Geometry check sheet. Reference: the model listing, model coordinates, mm. A direction names the side the tool comes from. Round coordinates to 2 decimals unless told otherwise and drop trailing zeros. Write each loop counter-clockwise with the first axis right and the second up, starting at its lowest first coordinate (ties: lowest second). Pieces come first, ordered by that corner, then holes.
Item 1: Access from +Z, -Z, +X, -X, +Y, -Y to the whole of each face (thin tool, end or side, straight path). Record for faces 1 (the face through (0, -115, 56)), 2 (the face through (3, -115, 54)).
Item 2: Cross-section at B-B (z = 31). Enter the section's corners in (x, y), then the cut area to 3 significant figures.
Item 3: Cross-section at A-A (y = -113.5). Enter the section's corners in (x, z).
Item 4: Cross-section at D-D (z = 52). Enter the section's corners in (x, y), then the cut area to 3 significant figures.
Item 5: Depth check by flat-ended pin: P1, Ø6, axis at x = 145, z = 97.5, coming from the +Y side; P2, Ø12, axis at x = 137, y = -119, coming from the -Z side. Enter the tip coordinate at first touch or a pass-through.
Item 6: Scan lines: probe 1 along Z at (x, y) = (2, -113.5); probe 2 along Y at (x, z) = (19.5, 89); probe 3 along X at (y, z) = (-25, 29). Record each from-to range of solid material in increasing order.
Item 7: Draft check along Z on faces 3 (the face through (98, 0, 54)), 4 (the face through (1.479, -102.444, 41.138)), 5 (the face through (98, -112, 110)). Enter one of: pulls with the +Z half, pulls with the -Z half, needs draft (parallel to the pull), parting line crosses it, or undercut.
Item 8: Cross-section at C-C (x = 154.5). Enter the section's corners in (y, z).
from build123d import *

# Parameters (mm, degrees)
F0_W     = 227
F0_H     = 110
F1_DEPTH = 3
F3_DEPTH = 195
F4_R     = 15
F5_DEPTH = 25


with BuildPart() as f1:
    # F0 (on Right) → F1 (new body)
    with BuildSketch(Plane.YZ):
        with Locations((-113.5, 55)):
            Rectangle(F0_W, F0_H)
    extrude(amount=F1_DEPTH)

    # F2 (on face) → F3 (join)
    with BuildSketch(Plane.YZ.offset(3)):
        Polygon((-3, 0), (0, 0), (0, 110), (-227, 110), (-227, 0), (-224, 0), (-224, 107), (-3, 107), align=None)
    extrude(amount=F3_DEPTH)

    # F4 (on face) → F5 (cut)
    with BuildSketch(Plane(origin=(0, 0, 0), x_dir=(0, -1, 0), z_dir=(-1, 0, 0))):
        with Locations((113.5, 31)):
            Circle(F4_R)
    extrude(amount=-F5_DEPTH, mode=Mode.SUBTRACT)


solid = f1.part
Resolved:
1. face 1: +Z, -Z, -X, +Y, -Y
1. face 2: -Z, +X
2. outline: (0, -227) - (198, -227) - (198, -224) - (3, -224) - (3, -128.5) - (0, -128.5) - close; (0, -98.5) - (3, -98.5) - (3, -3) - (198, -3) - (198, 0) - (0, 0) - close
2. area: 1,760 mm2
3. outline: (0, 0) - (3, 0) - (3, 16) - (0, 16) - close; (0, 46) - (3, 46) - (3, 107) - (198, 107) - (198, 110) - (0, 110) - close
4. outline: (0, -227) - (198, -227) - (198, -224) - (3, -224) - (3, -3) - (198, -3) - (198, 0) - (0, 0) - close
4. area: 1,850 mm2
5. P1: stops at y = 0
5. P2: stops at z = 107
6. probe 1: z = 0 to 16, 46 to 110
6. probe 2: y = -227 to -224, -3 to 0
6. probe 3: x = 0 to 3
7. face 3: needs draft
7. face 4: undercut
7. face 5: pulls with the +Z half
8. outline: (-227, 0) - (-224, 0) - (-224, 107) - (-3, 107) - (-3, 0) - (0, 0) - (0, 110) - (-227, 110) - close
